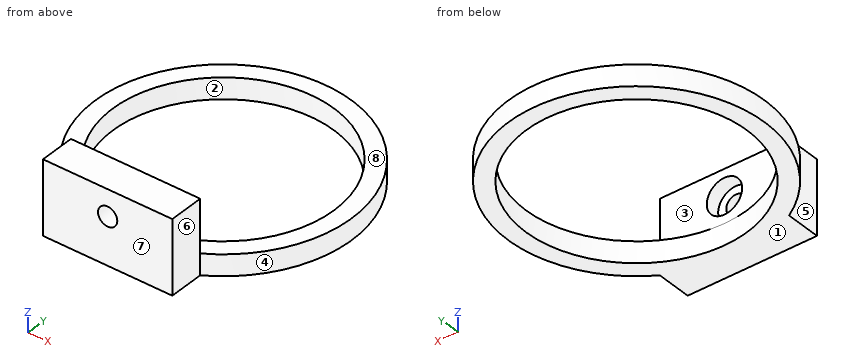
from build123d import *

# Parameters (mm, degrees)
SKETCH_R         = 31.5
PAD_DEPTH        = 6
SKETCH001_W      = 36.878178
SKETCH001_H      = 10
PAD001_DEPTH     = 15
HOLE_D           = 5.5
HOLE_DEPTH       = 25
HOLE_CBORE_D     = 10.1
HOLE_CBORE_DEPTH = 4.1


with BuildPart() as part:
    # Sketch → Pad (new body)
    with BuildSketch(Plane.XY):
        with BuildLine():
            ThreePointArc((18.439089, -31.5), (0, 36.5), (-18.439089, -31.5))
            Line((-18.439089, -31.5), (-18.439089, -41.5))
            Line((-18.439089, -41.5), (18.439089, -41.5))
            Line((18.439089, -41.5), (18.439089, -31.5))
        make_face()
        Circle(SKETCH_R, mode=Mode.SUBTRACT)
    extrude(amount=PAD_DEPTH)

    # Sketch001 (on Face7 of Pad) → Pad001 (join)
    with BuildSketch(Plane.XY.offset(6)):
        with Locations((0, -36.5)):
            Rectangle(SKETCH001_W, SKETCH001_H)
    extrude(amount=PAD001_DEPTH)

    # Hole
    with Locations(Plane(origin=(0, -31.5, 0), x_dir=(-1, 0, 0), z_dir=(0, 1, 0))):
        with Locations((0, 13.5)):
            CounterBoreHole(HOLE_D / 2, HOLE_CBORE_D / 2, HOLE_CBORE_DEPTH, depth=HOLE_DEPTH)


solid = part.part
For this review, take the finished solid that the model builds, in its own axes (mm). Face numbers are marked on the shaded views. A direction names the side the tool comes from. Coordinates: 2 decimals unless noted, no trailing zeros. Loops run counter-clockwise (first coordinate to the right, second up) from the corner with the lowest first, then second, coordinate; pieces in that order, holes last. Notation, with made-up numbers: (-8, 61.5) - (6, 61.5) arc R11 cw to (6, 65.5) - close; hole circle Ø11 at (44.5, -3.75). An arc over 180 degrees is marked (long way). Use a Markdown table: item, result. Add a question column.
Item 1: We need section C-C (x = 10.5). Give the boundary of the cut face in (y, z), and give its area (3 significant figures).
Item 2: For line 1 (Z direction, x = 0, y = -36.95); line 2 (Z direction, x = 0, y = -34.1); line 3 (X direction, y = 0, z = 1.25), list the stretches that pass through material, from the lowest coordinate up.
Item 3: Mouldability with a two-part tool opening along Y and no side actions: class the marked faces 1, 2, 3 and 4 as pulls with the +Y half, pulls with the -Y half, needs draft (parallel to the pull), parting line crosses it, or undercut.
Item 4: We need section A-A (y = 0). Give the boundary of the cut face in (x, z), and give its area (3 significant figures).
Item 5: Insertion check: pin 1 Ø8 at (y, z) = (-38, 7) entering from -X; pin 2 Ø8 at (y, z) = (-38.5, 10) entering from +X; pin 3 Ø1.5 at (y, z) = (24.5, 4.5) entering from -X. Each pin has a flat end and moves straight along its axis. Give the tip position at first contact, or say it passes through.
Item 6: Tool access review of the marked faces 5, 6, 7 and 8: name each direction out of +Z, -Z, +X, -X, +Y, -Y from which nothing blocks a thin tool from reaching the whole face with its end or side.
Item 7: We need section D-D (z = 3). Give the boundary of the cut face in (x, y), and give its area (3 significant figures).
Item 8: We need section B-B (z = 13.5). Give the boundary of the cut face in (x, y), and give its area (3 significant figures).
Results list:
| question | item | result |
|---|---|---|
| 1 | outline | (-41.5, 0) - (-29.7, 0) - (-29.7, 6) - (-31.5, 6) - (-31.5, 21) - (-41.5, 21) - close; (29.7, 0) - (34.96, 0) - (34.96, 6) - (29.7, 6) - close |
| 1 | area | 252 mm^2 |
| 2 | line 1 | z = 0 to 10.75, 16.25 to 21 |
| 2 | line 2 | z = 0 to 8.45, 18.55 to 21 |
| 2 | line 3 | x = -36.5 to -31.5, 31.5 to 36.5 |
| 3 | face 1 | needs draft |
| 3 | face 2 | undercut |
| 3 | face 3 | pulls with the +Y half |
| 3 | face 4 | parting line crosses it |
| 4 | outline | (-36.5, 0) - (-31.5, 0) - (-31.5, 6) - (-36.5, 6) - close; (31.5, 0) - (36.5, 0) - (36.5, 6) - (31.5, 6) - close |
| 4 | area | 60.0 mm^2 |
| 5 | pin 1 | stops at x = -18.44 |
| 5 | pin 2 | stops at x = 18.44 |
| 5 | pin 3 | stops at x = -27.72 |
| 6 | face 5 | +Z, -Z, -X, -Y |
| 6 | face 6 | +Z, -Z, +X, -Y |
| 6 | face 7 | +Z, -Z, +X, -X, -Y |
| 6 | face 8 | +Z, +X, -X, +Y |
| 7 | outline | (-18.44, -41.5) - (18.44, -41.5) - (18.44, -31.5) arc R36.5 ccw (long way) to (-18.44, -31.5) - close; hole circle Ø63 at (0, 0) |
| 7 | area | 1,310 mm^2 |
| 8 | outline | (-18.44, -41.5) - (-2.75, -41.5) - (-2.75, -35.6) - (-5.05, -35.6) - (-5.05, -31.5) - (-18.44, -31.5) - close; (2.75, -41.5) - (18.44, -41.5) - (18.44, -31.5) - (5.05, -31.5) - (5.05, -35.6) - (2.75, -35.6) - close |
| 8 | area | 295 mm^2 |
